```python
from build123d import *

# Parameters (mm, degrees)
ESQUISSE1_W             = 100
ESQUISSE1_H             = 30
BOSS_EXTRU_1_DEPTH      = 2
ESQUISSE2_W             = 2
ESQUISSE2_H             = 30
BOSS_EXTRU_2_DEPTH      = 70
ESQUISSE4_R             = 2
ENL_V_MAT_EXTRU_1_DEPTH = 101
CONG_1_R                = 1
CONG_2_R                = 1
ESQUISSE5_R             = 3
ENL_V_MAT_EXTRU_2_DEPTH = 10


with BuildPart() as part:
    # Esquisse1 → Boss.-Extru.1 (new body)
    with BuildSketch(Plane.XY):
        with Locations((50, -15)):
            Rectangle(ESQUISSE1_W, ESQUISSE1_H)
    extrude(amount=BOSS_EXTRU_1_DEPTH)

    # Esquisse2 → Boss.-Extru.2 (add)
    with BuildSketch(Plane.XY.offset(2)):
        with Locations((1, -15)):
            Rectangle(ESQUISSE2_W, ESQUISSE2_H)
    extrude(amount=BOSS_EXTRU_2_DEPTH)

    # Esquisse4 → Enlèv. mat.-Extru.1 (cut, through all)
    with BuildSketch(Plane.ZY):
        with Locations((52, -15)):
            Circle(ESQUISSE4_R)
    extrude(amount=-ENL_V_MAT_EXTRU_1_DEPTH, mode=Mode.SUBTRACT)

    # Congé1
    cong_1_edges = [part.edges().sort_by_distance(p)[0] for p in [
        (0, -15, 0),
    ]]
    fillet(cong_1_edges, radius=CONG_1_R)

    # Congé2
    cong_2_edges = [part.edges().sort_by_distance(p)[0] for p in [
        (100, -15, 0),
    ]]
    fillet(cong_2_edges, radius=CONG_2_R)

    # Esquisse5 → Enlèv. mat.-Extru.2 (cut)
    with BuildSketch(Plane(origin=(0, 0, 0), x_dir=(-1, 0, 0), z_dir=(0, 0, -1))):
        with Locations((-85, -15)):
            Circle(ESQUISSE5_R)
    extrude(amount=-ENL_V_MAT_EXTRU_2_DEPTH, mode=Mode.SUBTRACT)


solid = part.part
```
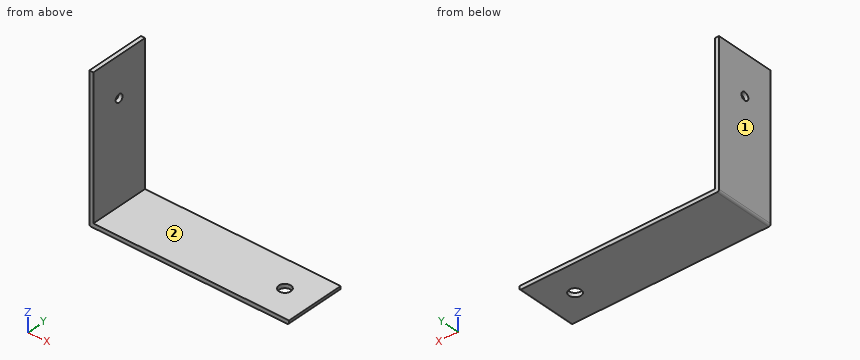
Here's how the part is built. I have some questions about the finished solid (model axes, mm). Face numbers are marked on the shaded views. A direction names the side the tool comes from. Give positions to 0.01 mm unless a question says otherwise; leave off trailing zeros. Write each loop counter-clockwise with the first axis right and the second up, starting at its lowest first coordinate (ties: lowest second). Pieces come first, ordered by that corner, then holes. Notation, with made-up numbers: (23.25, 21) -> (29.25, 21) arc R12 cw to (29.25, 31) -> close; hole circle Ø11 at (-12.5, -14). An arc over 180 degrees is marked (long way). Write each question's results on one line, items separated by ' | '.
Item 1: Suppose I cut it at B-B on x = 85. Write out the boundary of the cut face in (y, z).
Output:
outline: (-30, 0) -> (-18, 0) -> (-18, 2) -> (-30, 2) -> close; (-12, 0) -> (0, 0) -> (0, 2) -> (-12, 2) -> close
Item 2: If I drill on L1, parallel to Y at x = 1.6, z = 52; L2, parallel to Y at x = 85, z = 0.65; L3, parallel to X at y = -18.5, z = 53, over which ranges is the centre line in solid material (lowest first)?
Output:
L1: y = -30 to -17, -13 to 0 | L2: y = -30 to -18, -12 to 0 | L3: x = 0 to 2
Item 3: Suppose I cut it at D-D on y = -24.25. Write out the boundary of the cut face in (x, z).
Output:
outline: (0, 1) arc R1 ccw to (1, 0) -> (99, 0) arc R1 ccw to (100, 1) -> (100, 2) -> (2, 2) -> (2, 72) -> (0, 72) -> close
Item 4: Suppose I cut it at C-C on z = 52. Write out the boundary of the cut face in (x, y).
Output:
outline: (0, -30) -> (2, -30) -> (2, -17) -> (0, -17) -> close; (0, -13) -> (2, -13) -> (2, 0) -> (0, 0) -> close
Item 5: For pin 1 Ø15 at (y, z) = (-9, 54) entering from +X; pin 2 Ø5 at (x, y) = (85, -15) entering from +Z; pin 3 Ø1 at (x, y) = (61.5, -20.5) entering from +Z, each with a flat end and sliding along its axis, tell me the tip position at first contact or that it passes through.
Output:
pin 1: stops at x = 2 | pin 2: passes through | pin 3: stops at z = 2
Item 6: On a 3-axis mill with a long thin cutter (end or side, diameter ignored), from which of +Z, -Z, +X, -X, +Y, -Y can I reach the whole of each face in a straight line? I mean the marked faces 1 and 2. Say none if no direction works.
Output:
face 1: +Z, -Z, -X, +Y, -Y | face 2: +Z, +X, +Y, -Y
Item 7: Suppose I cut it at A-A on y = -15. Write out the boundary of the cut face in (x, z), plus the area to 3 significant figures.
Output:
outline: (0, 1) arc R1 ccw to (1, 0) -> (82, 0) -> (82, 2) -> (2, 2) -> (2, 50) -> (0, 50) -> close; (0, 54) -> (2, 54) -> (2, 72) -> (0, 72) -> close; (88, 0) -> (99, 0) arc R1 ccw to (100, 1) -> (100, 2) -> (88, 2) -> close | area: 320 mm^2
